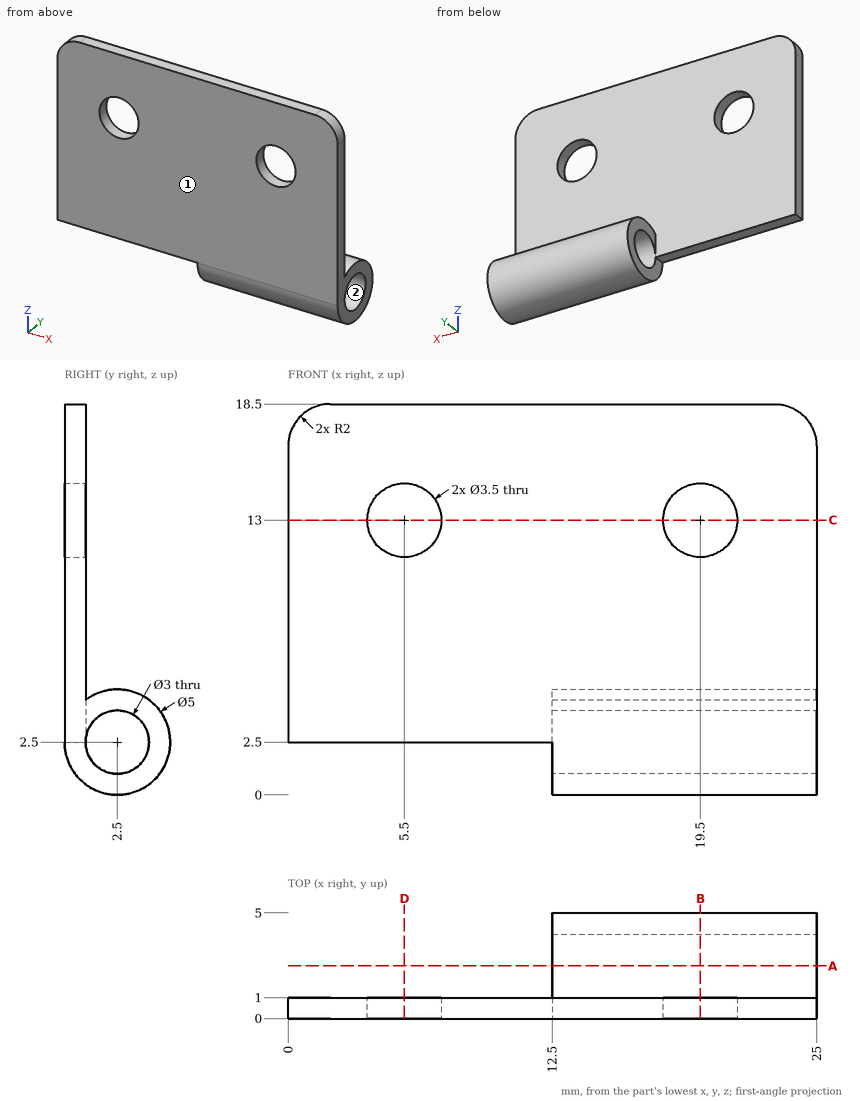
Can you work these out from the drawing? Everything is in mm from the part's minimum corner. Give positions to 0.01 mm unless a question says otherwise; leave off trailing zeros. Order: outer loops, then holes, each group sorted by start corner. A loop starts at its lowest first (then second) coordinate and runs counter-clockwise, first axis right, second up.
Item 1: If we section it at B-B, the plane x = 19.5: Write out the boundary of the cut face in (y, z), plus the area to 3 significant figures.
Item 2: If we section it at C-C, the plane z = 13: Write out the boundary of the cut face in (x, y), plus the area to 3 significant figures.
Item 3: I'm going to push flat-ended pins straight in: pin 1 (8 mm diameter, centred on x = 6.5, z = 11, fed in from +Y); pin 2 (3 mm diameter, centred on x = 7, z = 11.5, fed in from -Y); pin 3 (0.5 mm diameter, centred on x = 7.5, y = 0.5, fed in from -Z); pin 4 (3 mm diameter, centred on x = 13.5, y = 3.5, fed in from +Z). Where does each tip first touch, or does it pass through?
Item 4: If we mould it in two halves opening along Y, with no side actions, what happens to the marked faces 1 and 2? For each: pulls with the +Y half, pulls with the -Y half, needs draft (parallel to the pull), parting line crosses it, or undercut.
Item 5: If we section it at A-A, the plane y = 2.5: Write out the boundary of the cut face in (x, z).
Item 6: If we section it at D-D, the plane x = 5.5: Write out the boundary of the cut face in (y, z).
Item 7: I need wall thicknesses on line 1 (X direction, y = 0.5, z = 13); line 2 (Y direction, x = 21, z = 2.5). Which ranges of each line are inside material? Lowest first, please.
Values:
1. outline: (0, 2.5) arc R2.5 ccw (long way) to (1, 4.5) - (1, 11.25) - (0, 11.25) - close; (0, 14.75) - (1, 14.75) - (1, 18.5) - (0, 18.5) - close; hole circle Ø3 at (2.5, 2.5)
1. area: 23.7 mm2
2. outline: (0, 0) - (3.75, 0) - (3.75, 1) - (0, 1) - close; (7.25, 0) - (17.75, 0) - (17.75, 1) - (7.25, 1) - close; (21.25, 0) - (25, 0) - (25, 1) - (21.25, 1) - close
2. area: 18.0 mm2
3. pin 1: stops at y = 1
3. pin 2: stops at y = 0
3. pin 3: stops at z = 2.5
3. pin 4: stops at z = 5
4. face 1: pulls with the -Y half
4. face 2: undercut
5. outline: (12.5, 0) - (25, 0) - (25, 1) - (12.5, 1) - close; (12.5, 4) - (25, 4) - (25, 5) - (12.5, 5) - close
6. outline: (0, 2.5) - (1, 2.5) - (1, 11.25) - (0, 11.25) - close; (0, 14.75) - (1, 14.75) - (1, 18.5) - (0, 18.5) - close
7. line 1: x = 0 to 3.75, 7.25 to 17.75, 21.25 to 25
7. line 2: y = 0 to 1, 4 to 5
